from build123d import *

# Parameters (mm, degrees)
SKETCH_1_W             = 45
SKETCH_1_H             = 40
EXTRUDE_1_DEPTH        = 16
HOLE_WIZARD_M6_1_D     = 5
SKETCH_5_R             = 5.1
CUT_EXTRUDE_1_DEPTH    = 50
HOLE_WIZARD_M6_2_D     = 5
HOLE_WIZARD_M6_2_DEPTH = 10
HOLE_WIZARD_M6_2_TIP   = 1.502151548


with BuildPart() as part:
    # 草图1 → 凸台-拉伸1 (new body)
    with BuildSketch(Plane(origin=(0, 0, 0), x_dir=(1, 0, 0), z_dir=(0, 1, 0))):
        Rectangle(SKETCH_1_W, SKETCH_1_H)
    extrude(amount=EXTRUDE_1_DEPTH)

    # M6 螺纹孔1 (through all)
    with Locations(Plane(origin=(22.5, 8, 10), x_dir=(0, 0, 1), z_dir=(1, 0, 0))):
        with Locations((0, 0)):
            Hole(HOLE_WIZARD_M6_1_D / 2)

    # 草图5 → 切除-拉伸1 (cut)
    with BuildSketch(Plane(origin=(0, 16, 0), x_dir=(1, 0, 0), z_dir=(0, 1, 0))):
        with Locations(Location((10.5, 10, 0), (0, 0, 270))):
            Circle(SKETCH_5_R)
    extrude(amount=-CUT_EXTRUDE_1_DEPTH, mode=Mode.SUBTRACT)

    # M6 螺纹孔2
    with Locations(Plane(origin=(22.5, 8, -10), x_dir=(0, 0, 1), z_dir=(1, 0, 0))):
        with Locations((0, 0)):
            Hole(HOLE_WIZARD_M6_2_D / 2, depth=HOLE_WIZARD_M6_2_DEPTH)
            with Locations((0, 0, -(HOLE_WIZARD_M6_2_DEPTH + HOLE_WIZARD_M6_2_TIP / 2))):  # 118° drill point
                Cone(0, HOLE_WIZARD_M6_2_D / 2, HOLE_WIZARD_M6_2_TIP, mode=Mode.SUBTRACT)


solid = part.part
Geometry: final body of the model. Coordinates: model frame, mm. Coordinates: 2 decimals unless noted, no trailing zeros. Loops run counter-clockwise (first coordinate to the right, second up) from the corner with the lowest first, then second, coordinate; pieces in that order, holes last. Notation, with made-up numbers: M 87.25,-11.5 L 103.25,-11.5 A28 cw 103.25,20.5 Z; hole C -40,51 d3. An arc over 180 degrees is marked long. One line per item, written item: value. Start each with the question number.
1) Cut plane D-D (y = 7). Return loops of the section in (x, z), then the cut area to 3 significant figures.
2) Cut plane B-B (z = -10). Return loops of the section in (x, y).
3) Cut plane A-A (x = 10.5). Return loops of the section in (y, z).
4) Material intervals for L1, parallel to Z at x = 18.75, y = 8; L2, parallel to X at y = 4.5, z = -10; L3, parallel to Y at x = 2.5, z = 10, sorted ascending. Write a range as from..to.
5) Cut plane C-C (z = 10). Return loops of the section in (x, y).
6) Draft query along Z for faces 1 (the flat face through (0, 8, -20)), 2 (the cylindrical face through (18.7, 7.9, -7.5)), 3 (the flat face through (-22.5, 8, 0)). Return one class per face: released by +Z, released by -Z, zero draft, split by the parting line, or undercut.
Evaluation:
1. outline: M -22.5,-20 L 22.5,-20 L 22.5,-12.29 L 15.06,-12.29 A5.1 cw long 15.06,-7.71 L 22.5,-7.71 L 22.5,7.71 L -22.5,7.71 Z; M -22.5,12.29 L 22.5,12.29 L 22.5,20 L -22.5,20 Z
1. area: 1,480 mm^2
2. outline: M -22.5,0 L 5.4,0 L 5.4,16 L -22.5,16 Z; M 15.6,0 L 22.5,0 L 22.5,5.5 L 15.6,5.5 Z; M 15.6,10.5 L 22.5,10.5 L 22.5,16 L 15.6,16 Z
3. outline: M 0,-20 L 16,-20 L 16,-15.1 L 0,-15.1 Z; M 0,-4.9 L 16,-4.9 L 16,20 L 0,20 Z; hole C 8,10 d5
4. L1: -20..-12.5, -7.5..7.5, 12.5..20
4. L2: -22.5..5.4, 15.6..22.5
4. L3: 0..5.5, 10.5..16
5. outline: M -22.5,0 L 22.5,0 L 22.5,5.5 L -22.5,5.5 Z; M -22.5,10.5 L 22.5,10.5 L 22.5,16 L -22.5,16 Z
6. face 1: released by -Z
6. face 2: undercut
6. face 3: zero draft
